from build123d import *

# Parameters (mm, degrees)
EXTRUDE_1_DEPTH     = 1
CUT_EXTRUDE_1_REACH = 53.501
SKETCH_2_R          = 1.5
EXTRUDE_2_DEPTH     = 0.5


with BuildPart() as part:
    # 스케치1 → 보스-돌출1 (new body)
    with BuildSketch(Plane(origin=(0, 0, 0), x_dir=(1, 0, 0), z_dir=(0, 1, 0))):
        with BuildLine():
            Line((15.5, 47.342351167), (-2.051046792, 45.517737392))
            ThreePointArc((-2.051046792, 45.517737392), (-11.641492312, 40.641408305), (-15.5, 30.59814444))
            Line((-15.5, 30.59814444), (-15.5, -32.35898666))
            ThreePointArc((-15.5, -32.35898666), (-11.641492312, -42.402250525), (-2.051046792, -47.278579612))
            Line((-2.051046792, -47.278579612), (15.5, -49.103193387))
            Line((15.5, -49.103193387), (15.5, 47.342351167))
        make_face()
    extrude(amount=EXTRUDE_1_DEPTH)

    # 스케치2 → 컷-돌출1 (cut, up to next)
    with BuildSketch(Plane(origin=(0, 1, 0), x_dir=(1, 0, 0), z_dir=(0, 1, 0)), mode=Mode.PRIVATE) as cut_extrude_1_sk1:
        with Locations(Location((-1.637434314, 41.539179271, 0), (0, 0, 270))):
            Circle(SKETCH_2_R)
    cut_extrude_1_tool1 = extrude(cut_extrude_1_sk1.sketch, amount=-CUT_EXTRUDE_1_REACH, mode=Mode.PRIVATE) & part.part
    # 스케치2 → 컷-돌출1 (cut, up to next)
    with BuildSketch(Plane(origin=(0, 1, 0), x_dir=(1, 0, 0), z_dir=(0, 1, 0)), mode=Mode.PRIVATE) as cut_extrude_1_sk2:
        with Locations(Location((-11.5, 17.694952146, 0), (0, 0, 270))):
            Circle(SKETCH_2_R)
    cut_extrude_1_tool2 = extrude(cut_extrude_1_sk2.sketch, amount=-CUT_EXTRUDE_1_REACH, mode=Mode.PRIVATE) & part.part
    # 스케치2 → 컷-돌출1 (cut, up to next)
    with BuildSketch(Plane(origin=(0, 1, 0), x_dir=(1, 0, 0), z_dir=(0, 1, 0)), mode=Mode.PRIVATE) as cut_extrude_1_sk3:
        with Locations(Location((-11.5, -19.455794366, 0), (0, 0, 270))):
            Circle(SKETCH_2_R)
    cut_extrude_1_tool3 = extrude(cut_extrude_1_sk3.sketch, amount=-CUT_EXTRUDE_1_REACH, mode=Mode.PRIVATE) & part.part
    # 스케치2 → 컷-돌출1 (cut, up to next)
    with BuildSketch(Plane(origin=(0, 1, 0), x_dir=(1, 0, 0), z_dir=(0, 1, 0)), mode=Mode.PRIVATE) as cut_extrude_1_sk4:
        with Locations(Location((-1.637434314, -43.300021491, 0), (0, 0, 270))):
            Circle(SKETCH_2_R)
    cut_extrude_1_tool4 = extrude(cut_extrude_1_sk4.sketch, amount=-CUT_EXTRUDE_1_REACH, mode=Mode.PRIVATE) & part.part
    # 스케치2 → 컷-돌출1 (cut, up to next)
    with BuildSketch(Plane(origin=(0, 1, 0), x_dir=(1, 0, 0), z_dir=(0, 1, 0)), mode=Mode.PRIVATE) as cut_extrude_1_sk5:
        with Locations(Location((12.5, 29.11957889, 0), (0, 0, 270))):
            Circle(SKETCH_2_R)
    cut_extrude_1_tool5 = extrude(cut_extrude_1_sk5.sketch, amount=-CUT_EXTRUDE_1_REACH, mode=Mode.PRIVATE) & part.part
    # 스케치2 → 컷-돌출1 (cut, up to next)
    with BuildSketch(Plane(origin=(0, 1, 0), x_dir=(1, 0, 0), z_dir=(0, 1, 0)), mode=Mode.PRIVATE) as cut_extrude_1_sk6:
        with Locations(Location((12.5, -30.88042111, 0), (0, 0, 270))):
            Circle(SKETCH_2_R)
    cut_extrude_1_tool6 = extrude(cut_extrude_1_sk6.sketch, amount=-CUT_EXTRUDE_1_REACH, mode=Mode.PRIVATE) & part.part
    add(cut_extrude_1_tool1.solids().sort_by_distance((-1.637434, 1, -41.539179))[0], mode=Mode.SUBTRACT)
    add(cut_extrude_1_tool2.solids().sort_by_distance((-11.5, 1, -17.694952))[0], mode=Mode.SUBTRACT)
    add(cut_extrude_1_tool3.solids().sort_by_distance((-11.5, 1, 19.455794))[0], mode=Mode.SUBTRACT)
    add(cut_extrude_1_tool4.solids().sort_by_distance((-1.637434, 1, 43.300021))[0], mode=Mode.SUBTRACT)
    add(cut_extrude_1_tool5.solids().sort_by_distance((12.5, 1, -29.119579))[0], mode=Mode.SUBTRACT)
    add(cut_extrude_1_tool6.solids().sort_by_distance((12.5, 1, 30.880421))[0], mode=Mode.SUBTRACT)

    # 스케치3 → 보스-돌출2 (add)
    with BuildSketch(Plane.XZ):
        with BuildLine():
            Line((-11.3, -14.952234515), (-11.3, 16.713076735))
            ThreePointArc((-11.3, 16.713076735), (-8.75, 19.455794366), (-11.3, 22.198511996))
            Line((-11.3, 22.198511996), (-11.3, 32.35898666))
            ThreePointArc((-11.3, 32.35898666), (-9.367936379, 38.523376685), (-4.263017708, 42.482212318))
            ThreePointArc((-4.263017708, 42.482212318), (-1.182011658, 40.587994536), (1.111261685, 43.384699144))
            Line((1.111261685, 43.384699144), (9.3, 44.236003622))
            Line((9.3, 44.236003622), (9.3, -42.475161402))
            Line((9.3, -42.475161402), (1.111261685, -41.623856924))
            ThreePointArc((1.111261685, -41.623856924), (-1.182011658, -38.827152317), (-4.263017708, -40.721370098))
            ThreePointArc((-4.263017708, -40.721370098), (-9.367936379, -36.762534465), (-11.3, -30.59814444))
            Line((-11.3, -30.59814444), (-11.3, -20.437669776))
            ThreePointArc((-11.3, -20.437669776), (-8.75, -17.694952146), (-11.3, -14.952234515))
        make_face()
    extrude(amount=EXTRUDE_2_DEPTH)


solid = part.part
Verification items for the finished model (mm, model axes). A direction names the side the tool comes from. Give positions to 0.01 mm unless a question says otherwise; leave off trailing zeros. Write each loop counter-clockwise with the first axis right and the second up, starting at its lowest first coordinate (ties: lowest second). Pieces come first, ordered by that corner, then holes. Notation, with made-up numbers: M 33,29 L 92,29 A23 cw 92,56 Z; hole C -6,69 d2. An arc over 180 degrees is marked long. Put each result on its own line as item: value. Start each with the question number.
1. Section check A-A (z = -29.5). Record the cut outline in (x, y).
2. Go/stop test with a flat-tipped pin: pin 1 Ø4 at (x, z) = (-11.5, -17.69) entering from -Y. Record where the tip stops, or that it passes through.
3. Section check D-D (y = 0.7). Record the cut outline in (x, z), and give its area (3 significant figures).
4. Set-up check for faces 4 (the face through (-11.74, 0.49, 42.29)), 5 (the face through (-9.315, -0.246, -36.838)), 6 (the face through (-8.75, -0.25, 19.4)): record each of +Z, -Z, +X, -X, +Y, -Y from which the full face is reachable in a straight line by a thin tool's end or side.
5. Section check B-B (x = 12.5). Record the cut outline in (y, z).
6. Scan lines: line 1 along Z through (x, y) = (-1, 0.4); line 2 along X through (y, z) = (0.55, 33); line 3 along Y through (x, z) = (11, 21.5). Record each from-to range of solid material in increasing order. Write a range as [from, to].
7. Draft check along X on faces 1 (the face through (-1, -0.5, 1)), 2 (the face through (-2.55, 0.51, 42.11)), 3 (the face through (-9.42, -0.25, 38.45)). Enter one of: +X half, -X half, draft (parallel to the pull), parting line (faces both ways), or undercut.
8. Section check C-C (z = -3). Record the cut outline in (x, y).
Answer list:
1. outline: M -15.5,0 L -11.3,0 L -11.3,-0.5 L 9.3,-0.5 L 9.3,0 L 11.05,0 L 11.05,1 L -15.5,1 Z; M 13.95,0 L 15.5,0 L 15.5,1 L 13.95,1 Z
2. pin 1: y = 0
3. outline: M -15.5,-30.6 A15 ccw -2.05,-45.52 L 15.5,-47.34 L 15.5,49.1 L -2.05,47.28 A15 ccw -15.5,32.36 Z; hole C -11.5,-17.69 d3; hole C -11.5,19.46 d3; hole C -1.64,-41.54 d3; hole C -1.64,43.3 d3; hole C 12.5,-29.12 d3; hole C 12.5,30.88 d3
3. area: 2,770 mm2
4. face 4: +Z, -X, +Y, -Y
4. face 5: -Z, -X, -Y
4. face 6: -X, -Y
5. outline: M 0,-47.03 L 1,-47.03 L 1,-30.62 L 0,-30.62 Z; M 0,-27.62 L 1,-27.62 L 1,29.38 L 0,29.38 Z; M 0,32.38 L 1,32.38 L 1,48.79 L 0,48.79 Z
6. line 1: [-45.63, -42.9], [-40.18, 41.94], [44.66, 47.39]
6. line 2: [-15.49, 15.5]
6. line 3: [0, 1]
7. face 1: draft
7. face 2: undercut
7. face 3: -X half
8. outline: M -15.5,0 L -11.3,0 L -11.3,-0.5 L 9.3,-0.5 L 9.3,0 L 15.5,0 L 15.5,1 L -15.5,1 Z
